from build123d import *

# Parameters (mm, degrees)
CROQUIS1_W              = 530
CROQUIS1_H              = 1200
CROQUIS1_W_2            = 500
CROQUIS1_H_2            = 1170
SALIENTE_EXTRUIR1_DEPTH = 15
REDONDEO1_R             = 2
REDONDEO2_R             = 2
CROQUIS2_R              = 3.75
SALIENTE_EXTRUIR2_DEPTH = 15
CROQUIS3_R              = 5
CORTAR_EXTRUIR1_DEPTH   = 546
CROQUIS4_R              = 3.75
SALIENTE_EXTRUIR3_DEPTH = 30
CROQUIS5_R              = 3.75
SALIENTE_EXTRUIR4_DEPTH = 30
ESCALA1_SCALE           = 1.3


with BuildPart() as part:
    # Croquis1 → Saliente-Extruir1 (new body)
    with BuildSketch(Plane(origin=(0, 0, 0), x_dir=(1, 0, 0), z_dir=(0, 1, 0))):
        Rectangle(CROQUIS1_W, CROQUIS1_H)
        Rectangle(CROQUIS1_W_2, CROQUIS1_H_2, mode=Mode.SUBTRACT)
    extrude(amount=SALIENTE_EXTRUIR1_DEPTH)

    # Redondeo1
    redondeo1_edges = [part.edges().sort_by_distance(p)[0] for p in [
        (-265, 15, 0),
        (250, 15, 0),
        (0, 15, 600),
        (0, 15, -585),
        (-250, 15, 0),
        (0, 15, 585),
        (265, 15, 0),
        (0, 15, -600),
    ]]
    fillet(redondeo1_edges, radius=REDONDEO1_R)

    # Redondeo2
    redondeo2_edges = [part.edges().sort_by_distance(p)[0] for p in [
        (250, 0, 0),
        (0, 0, -585),
        (-250, 0, 0),
        (0, 0, 585),
        (0, 0, 600),
        (-265, 0, 0),
        (0, 0, -600),
        (265, 0, 0),
    ]]
    fillet(redondeo2_edges, radius=REDONDEO2_R)

    # Croquis2 → Saliente-Extruir2 (add)
    with BuildSketch(Plane.ZY.offset(265)):
        with Locations((596.25, 7.5)):
            Circle(CROQUIS2_R)
        with Locations((-596.25, 7.5)):
            Circle(CROQUIS2_R)
    saliente_extruir2 = extrude(amount=SALIENTE_EXTRUIR2_DEPTH)

    # Simetría1: Saliente-Extruir2 across plane
    add(saliente_extruir2.mirror(Plane(origin=(0, 0, 0), x_dir=(0, 0, 1), z_dir=(1, 0, 0))))

    # Croquis3 → Cortar-Extruir1 (cut, through all)
    with BuildSketch(Plane.ZY.offset(265)):
        with Locations((0, 7.5)):
            Circle(CROQUIS3_R)
    extrude(amount=-CORTAR_EXTRUIR1_DEPTH, mode=Mode.SUBTRACT)

    # Croquis4 → Saliente-Extruir3 (add)
    with BuildSketch(Plane(origin=(280, 0, 0), x_dir=(0, 0, -1), z_dir=(1, 0, 0))):
        with Locations((-596.25, 7.5)):
            Circle(CROQUIS4_R)
    extrude(amount=SALIENTE_EXTRUIR3_DEPTH)

    # Croquis5 → Saliente-Extruir4 (add)
    with BuildSketch(Plane.ZY.offset(280)):
        with Locations((596.25, 7.5)):
            Circle(CROQUIS5_R)
    extrude(amount=SALIENTE_EXTRUIR4_DEPTH)


with BuildPart() as part_1:
    # Escala1: scaled about (0, 0, 0)
    add(part.part.scale(ESCALA1_SCALE))


solid = part_1.part
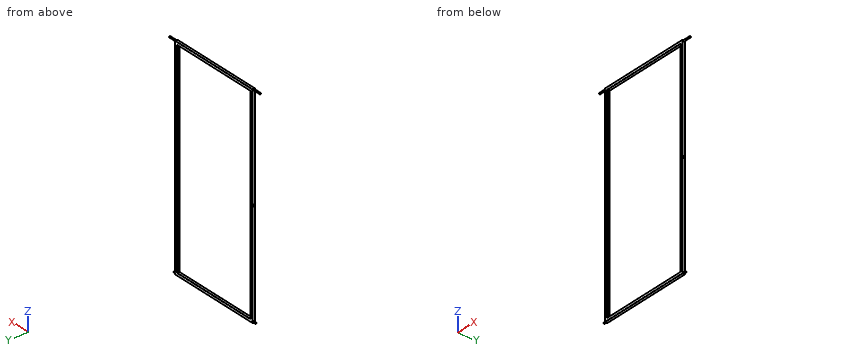
The model under review builds one solid part; all positions refer to its coordinate system, in mm. Give positions to 0.01 mm unless a question says otherwise; leave off trailing zeros. Write each loop counter-clockwise with the first axis right and the second up, starting at its lowest first coordinate (ties: lowest second). Pieces come first, ordered by that corner, then holes.
1. Add section B-B, the plane z = -173.5. Write out the cut boundary in (x, y), plus the area to 3 significant figures.
2. Add section A-A, the plane x = -51.5. Write out the cut boundary in (y, z).
3. Wall thickness on L1, parallel to X at y = 13.5, z = 157.5; L2, parallel to Y at x = -331, z = 0; L3, parallel to Z at x = 74, y = 16.5: over which ranges is each line inside the solid? List them lowest first.
4. For P1, Ø6, axis at y = 6, z = 433.5, coming from the -X side; P2, Ø3, axis at y = 11.5, z = -775, coming from the -X side; P3, Ø10, axis at y = 8.5, z = -51.5, coming from the +X side, all flat-tipped, find the tip position at first contact; note any pin that passes through.
Worked answers:
1. outline: (-344.5, 2.6) arc R2.6 ccw to (-341.9, 0) - (-327.6, 0) arc R2.6 ccw to (-325, 2.6) - (-325, 16.9) arc R2.6 ccw to (-327.6, 19.5) - (-341.9, 19.5) arc R2.6 ccw to (-344.5, 16.9) - close; (325, 2.6) arc R2.6 ccw to (327.6, 0) - (341.9, 0) arc R2.6 ccw to (344.5, 2.6) - (344.5, 16.9) arc R2.6 ccw to (341.9, 19.5) - (327.6, 19.5) arc R2.6 ccw to (325, 16.9) - close
1. area: 749 mm2
2. outline: (0, -777.4) arc R2.6 ccw to (2.6, -780) - (16.9, -780) arc R2.6 ccw to (19.5, -777.4) - (19.5, -763.1) arc R2.6 ccw to (16.9, -760.5) - (2.6, -760.5) arc R2.6 ccw to (0, -763.1) - close; (0, 763.1) arc R2.6 ccw to (2.6, 760.5) - (16.9, 760.5) arc R2.6 ccw to (19.5, 763.1) - (19.5, 777.4) arc R2.6 ccw to (16.9, 780) - (2.6, 780) arc R2.6 ccw to (0, 777.4) - close
3. L1: x = -344.5 to -325, 325 to 344.5
3. L2: y = 0 to 3.25, 16.25 to 19.5
3. L3: z = -780 to -760.5, 760.5 to 780
4. P1: stops at x = -344.5
4. P2: stops at x = -364
4. P3: stops at x = 344.5
